Part model, mm, in its own coordinate system. Face numbers are marked on the shaded views. A direction names the side the tool comes from. Give positions to 0.01 mm unless a question says otherwise; leave off trailing zeros. Order: outer loops, then holes, each group sorted by start corner. A loop starts at its lowest first (then second) coordinate and runs counter-clockwise, first axis right, second up. Notation, with made-up numbers: M 39,8 L 51,8 A22 cw 51,34 Z; hole C 37,8.25 d7. An arc over 180 degrees is marked long. Answer as a JSON object with one key per item and string values.
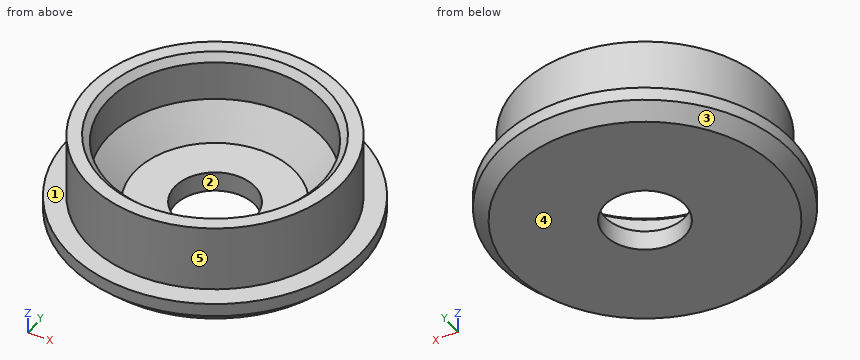
Autodesk Inventor part; units mm, degrees
ref_plane "YZ Plane" through (0, 0, 0) normal (1, 0, 0) x (0, 1, 0)
ref_plane "XZ Plane" through (0, 0, 0) normal (0, 1, 0) x (-1, 0, 0)
ref_plane "XY Plane" through (0, 0, 0) normal (0, 0, 1) x (1, 0, 0)
sketch "Esquisse1" plane through (0, 0, 0) normal (1, 0, 0) x (0, 1, 0)
  line L0 (22, 4) -> (22, 0)
  line L1 (22, 4) -> (19, 4)
  line L2 (19, 4) -> (19, 14)
  line L3 (19, 14) -> (16, 14)
  line L4 (16, 14) -> (16, 3)
  line L5 (22, 0) -> (6, 0)
  line L6 (6, 0) -> (6, 3)
  line L7 (6, 3) -> (16, 3)
  line L8 (0, 0) -> (0, -5.3906)
  dimension "d0" = 4
  dimension "d2" = 10
  dimension "d3" = 3
  dimension "d4" = 12
  dimension "d7" = 38
  dimension "d8" = 3
  dimension "d9" = 3
revolve "Révolution1" add sketch "Esquisse1" angle 360 about axis through (0, 0, 0) along (0, 0, -1)
chamfer "Chanfrein1" distance 2 angle 45 1 edges at (0, -22, 0)
chamfer "Chanfrein2" distance 4 angle 45 1 edges at (0, -16, 3)
thread "Filetage1"
chamfer "Chanfrein3" distance 1 angle 45 1 edges at (0, -16, 14)
thread "Filetage2"
properties part number "reservoir_cullasse"
1. Cut at A-A on y = 0. Give the cut face in (x, z).
Worked answers:
{"outline": "M -22,2 L -20,0 L -6,0 L -6,3 L -12,3 L -16,7 L -16,13 L -17,14 L -19,14 L -19,4 L -22,4 Z; M 6,0 L 20,0 L 22,2 L 22,4 L 19,4 L 19,14 L 17,14 L 16,13 L 16,7 L 12,3 L 6,3 Z"}
2. Cut at C-C on z = 10. Give the cut face in (x, y).
Worked answers:
{"outline": "C 0,0 d38; hole C 0,0 d32"}
3. Probe line 1 along X through (y, z) = (0, 2.15); line 2 along X through (y, z) = (-0.5, 7); line 3 along Y through (x, z) = (-3, 7.25). List the from-to ranges inside material, lowest first.
Worked answers:
{"line 1": "x = -22 to -6, 6 to 22", "line 2": "x = -18.99 to -15.99, 15.99 to 18.99", "line 3": "y = -18.76 to -15.72, 15.72 to 18.76"}
4. Which spindle directions (+Z, -Z, +X, -X, +Y, -Y) get a long thin tool onto all of the face, cutting with end or side? Do the marked faces 4 and 5. Say none if no direction does.
Worked answers:
{"face 4": "-Z, +X, -X, +Y, -Y", "face 5": "+Z"}
5. Cut at B-B on z = 5.75. Give the cut face in (x, y), plus the area to 3 significant figures.
Worked answers:
{"outline": "C 0,0 d38; hole C 0,0 d29.5", "area": "451 mm^2"}
6. Pin check, flat tips, straight feed: P1, Ø1.5, axis at x = 8, z = 6, coming from the -Y side; P2, Ø2, axis at x = -3.5, y = 8.5, coming from the -Z side; P3, Ø5, axis at y = -14.5, z = 5.5, coming from the -X side; P4, Ø3, axis at y = -17, z = 11.5, coming from the +X side. Stop position of each tip, or through.
Worked answers:
{"P1": "stops at y = -17.56", "P2": "stops at z = 0", "P3": "stops at x = -18.1", "P4": "stops at x = 10.99"}
7. Two-plate mould, pull along Y, no slides. Class the marked faces 1, 2 and 3: +Y half, -Y half, draft (parallel to the pull), parting line (faces both ways), or undercut.
Worked answers:
{"face 1": "draft", "face 2": "undercut", "face 3": "parting line"}
